Job drawing, mm, ordinate dimensions from the low corner. One solid piece. A direction names the side the tool comes from. Give positions to 0.01 mm unless a question says otherwise; leave off trailing zeros. Order: outer loops, then holes, each group sorted by start corner. A loop starts at its lowest first (then second) coordinate and runs counter-clockwise, first axis right, second up. Notation, with made-up numbers: (58, 82.5) - (85, 82.5) arc R24 cw to (85, 92.5) - close; hole circle Ø9 at (-14.75, -15.75). An arc over 180 degrees is marked (long way). Use one line per item in the form item = value. Start each with the question number.
1. Tool access for the marked faces 5, 6 and 7: list every direction of +Z, -Z, +X, -X, +Y, -Y with a clear straight run to the whole face (end or side of a thin tool).
2. Band-saw the part on C-C, the plane z = 3.5. List the corners of the cut face in (x, y) (1 decimal).
3. Band-saw the part on B-B, the plane y = 6.75. List the corners of the cut face in (x, z).
4. Drill centre lines: line 1 (X direction, y = 8.25, z = 4.75); line 2 (Z direction, x = 15.5, y = 9); line 3 (Y direction, x = 4.75, z = 19.75). Where is each one in solid material? Low to high.
5. Band-saw the part on D-D, the plane z = 14. List the corners of the cut face in (x, y).
6. Band-saw the part on A-A, the plane x = 19.93. List the corners of the cut face in (y, z) (1 decimal).
7. Pull direction X, two halves, no side cores. Call the marked faces 1, 2, 3 and 4: +X half, -X half, draft (parallel to the pull), parting line (faces both ways), or undercut.
8. Pin check, flat tips, straight feed: P1, Ø4, axis at y = 7.5, z = 3.5, coming from the -X side; P2, Ø1, axis at y = 5, z = 18, coming from the +X side; P3, Ø1.4, axis at x = 10.5, z = 1.5, coming from the -Y side; P4, Ø2, axis at x = 19.93, z = 17.72, coming from the +Y side. Stop position of each tip, or through.
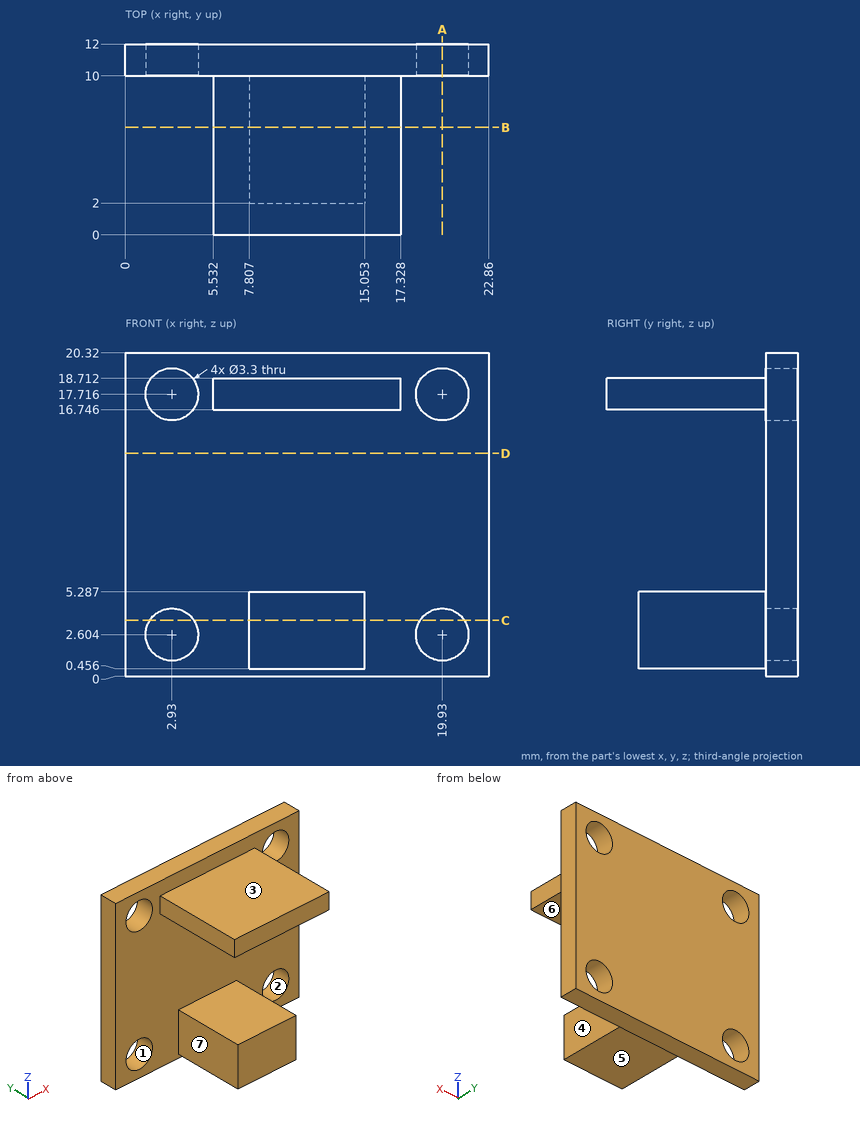
From the geometry:
q1.face_5 = -Z, +X, -X, -Y
q1.face_6 = +X, -X, -Y
q1.face_7 = -Z, -X, -Y
q2.outline = (0, 10) - (1.5, 10) - (1.5, 12) - (0, 12) - close; (4.3, 10) - (7.8, 10) - (7.8, 2) - (15.1, 2) - (15.1, 10) - (18.5, 10) - (18.5, 12) - (4.3, 12) - close; (21.3, 10) - (22.9, 10) - (22.9, 12) - (21.3, 12) - close
q3.outline = (5.53, 16.75) - (17.33, 16.75) - (17.33, 18.71) - (5.53, 18.71) - close; (7.81, 0.46) - (15.05, 0.46) - (15.05, 5.29) - (7.81, 5.29) - close
q4.line_1 = 7.81 to 15.05
q4.line_2 = 16.75 to 18.71
q4.line_3 = 10 to 12
q5.outline = (0, 10) - (22.86, 10) - (22.86, 12) - (0, 12) - close
q6.outline = (10, 0) - (12, 0) - (12, 1) - (10, 1) - close; (10, 4.3) - (12, 4.3) - (12, 16.1) - (10, 16.1) - close; (10, 19.4) - (12, 19.4) - (12, 20.3) - (10, 20.3) - close
q7.face_1 = undercut
q7.face_2 = undercut
q7.face_3 = draft
q7.face_4 = +X half
q8.P1 = 7.81
q8.P2 = 17.33
q8.P3 = 2
q8.P4 = through
